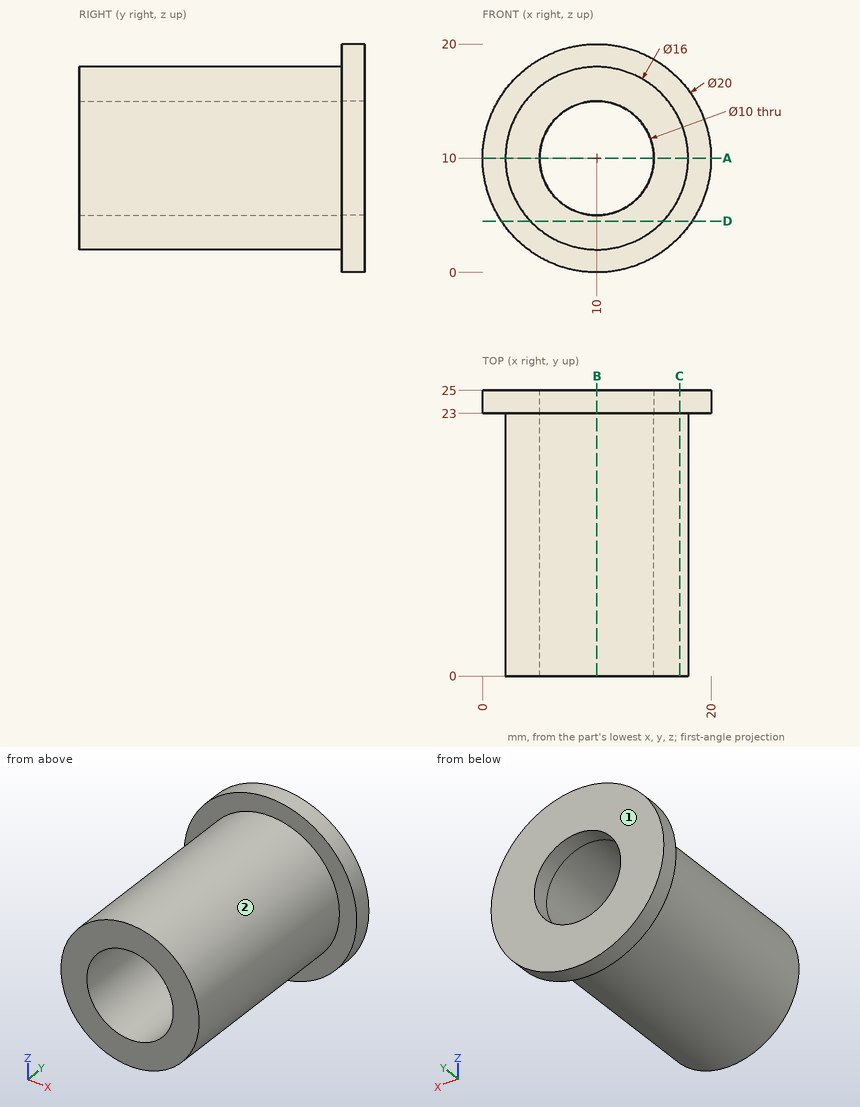
Can you work these out from the drawing? Everything is in mm from the part's minimum corner. A direction names the side the tool comes from. Round coordinates to 2 decimals unless told otherwise and drop trailing zeros. Loops run counter-clockwise (first coordinate to the right, second up) from the corner with the lowest first, then second, coordinate; pieces in that order, holes last.
1. If we section it at A-A on z = 10: Write out the boundary of the cut face in (x, y), plus the area to 3 significant figures.
Answer list:
outline: (0, 23) - (2, 23) - (2, 0) - (5, 0) - (5, 25) - (0, 25) - close; (15, 0) - (18, 0) - (18, 23) - (20, 23) - (20, 25) - (15, 25) - close
area: 158 mm2
2. For P1, Ø3, axis at x = 10.5, y = 14, coming from the -Z side; P2, Ø1.5, axis at x = 11.5, y = 20.5, coming from the +Z side; P3, Ø9, axis at x = 10, z = 10, coming from the +Y side; P4, Ø6, axis at y = 12.5, z = 2.5, coming from the +X side, each with a flat end and sliding along its axis, tell me the tip position at first contact or that it passes through.
Answer list:
P1: stops at z = 2
P2: stops at z = 17.96
P3: passes through
P4: stops at x = 16.61
3. Which directions (+Z, -Z, +X, -X, +Y, -Y) give clear straight access to the entire face, cutting with the end or side of a thin tool? Please do the marked faces 1 and 2.
Answer list:
face 1: +Z, -Z, +X, -X, +Y
face 2: -Y
4. If we section it at D-D on z = 4.5: Write out the boundary of the cut face in (x, y).
Answer list:
outline: (1.65, 23) - (4.19, 23) - (4.19, 0) - (15.81, 0) - (15.81, 23) - (18.35, 23) - (18.35, 25) - (1.65, 25) - close
5. If we section it at C-C on x = 17.25: Write out the boundary of the cut face in (y, z).
Answer list:
outline: (0, 6.62) - (23, 6.62) - (23, 3.11) - (25, 3.11) - (25, 16.89) - (23, 16.89) - (23, 13.38) - (0, 13.38) - close
6. If we section it at B-B on x = 10: Write out the boundary of the cut face in (y, z), plus the area to 3 significant figures.
Answer list:
outline: (0, 2) - (23, 2) - (23, 0) - (25, 0) - (25, 5) - (0, 5) - close; (0, 15) - (25, 15) - (25, 20) - (23, 20) - (23, 18) - (0, 18) - close
area: 158 mm2
7. If I drill on line 1 along Z through (x, y) = (10, 5.25); line 2 along Y through (x, z) = (1.5, 7.25); line 3 along X through (y, z) = (23.75, 10.25), over which ranges is the centre line in solid material (lowest first)?
Answer list:
line 1: z = 2 to 5, 15 to 18
line 2: y = 23 to 25
line 3: x = 0 to 5.01, 14.99 to 20
